The model under review builds one solid part; all positions refer to its coordinate system, in mm. A direction names the side the tool comes from. Round coordinates to 2 decimals unless told otherwise and drop trailing zeros. Write each loop counter-clockwise with the first axis right and the second up, starting at its lowest first coordinate (ties: lowest second). Pieces come first, ordered by that corner, then holes. Notation, with made-up numbers: (36, 83) -> (61, 83) arc R30 cw to (61, 121) -> close; hole circle Ø8 at (5.5, 86.5). An arc over 180 degrees is marked (long way). Return JSON: item names as keys, results as strings. Group by question number.
1. Take a section at A-A, the plane y = 15. Write out the cut boundary in (x, z).
2. For line 1 along X through (y, z) = (16.25, 0.5); line 2 along Z through (x, y) = (6.75, 18); line 3 along X through (y, z) = (8, -4.5), list the stretches that pass through material, from the lowest coordinate up. Write a range as from..to.
3. Take a section at B-B, the plane z = 0.25. Write out the cut boundary in (x, y), then the cut area to 3 significant figures.
4. Mouldability with a two-part tool opening along Y and no side actions: class faces 1 (the flat face through (2, 0, -1)), 2 (the flat face through (2, 20, -1)), 3 (the flat face through (6.252, 10, 2)) as pulls with the +Y half, pulls with the -Y half, needs draft (parallel to the pull), parting line crosses it, or undercut.
5. Clearance check with flat-ended pins moving along their axes: P1, Ø2, axis at y = 9, z = 3, coming from the -X side; P2, Ø2, axis at x = 8, y = 10.5, coming from the +Z side. State where each tip first meets the part, or that it passes through.
6. Take a section at C-C, the plane x = 9. Write out the cut boundary in (y, z), then the cut area to 3 significant figures.
7. Tool access review of faces 4 (the flat face through (8, 10, 0)), 5 (the flat face through (-1.748, 10, 2)), 6 (the flat face through (2, 10, -6.46)): name each direction out of +Z, -Z, +X, -X, +Y, -Y from which nothing blocks a thin tool from reaching the whole face with its end or side.
from build123d import *

# Parameters (mm, degrees)
BOSS_EXTRUDE1_DEPTH          = 40
SKETCH2_W                    = 3.5
SKETCH2_H                    = 40
BOSS_EXTRUDE2_DEPTH          = 5
SKETCH4_R                    = 2
CUT_EXTRUDE1_DEPTH           = 7
SKETCH5_R                    = 3.5
CUT_EXTRUDE2_DEPTH           = 3
CUT_EXTRUDE2_DRAFT           = -27
CUT_EXTRUDE2_PROFILE_2_DEPTH = 3
CUT_EXTRUDE2_PROFILE_2_DRAFT = -27
BOSS_EXTRUDE3_DEPTH          = 3
SKETCH9_W                    = 13
SKETCH9_H                    = 40
CUT_EXTRUDE4_DEPTH           = 4.702585656
SKETCH10_W                   = 15
SKETCH10_H                   = 40
BOSS_EXTRUDE4_DEPTH          = 2.5
SKETCH11_W                   = 1.5
SKETCH11_H                   = 2.202585656
BOSS_EXTRUDE7_DEPTH          = 40
BOSS_EXTRUDE8_DEPTH          = 0.625841469
SKETCH13_R                   = 2
CUT_EXTRUDE5_DEPTH           = 10
SKETCH14_W                   = 2.5
SKETCH14_H                   = 40
BOSS_EXTRUDE9_DEPTH          = 0.5
SKETCH15_W                   = 2.5
SKETCH15_H                   = 40
BOSS_EXTRUDE10_DEPTH         = 0.5
BOSS_EXTRUDE11_DEPTH         = 40
BOSS_EXTRUDE12_DEPTH         = 1.13137085
SKETCH18_R                   = 2
CUT_EXTRUDE6_DEPTH           = 10
SKETCH19_R                   = 3
CUT_EXTRUDE7_DEPTH           = 3
CUT_EXTRUDE7_DRAFT           = -19
CUT_EXTRUDE7_PROFILE_2_DEPTH = 3
CUT_EXTRUDE7_PROFILE_2_DRAFT = -19
SKETCH20_W                   = 5
SKETCH20_H                   = 40
BOSS_EXTRUDE13_DEPTH         = 0.5
SKETCH21_W                   = 5
SKETCH21_H                   = 40
BOSS_EXTRUDE14_DEPTH         = 0.5
SKETCH22_W                   = 7
SKETCH22_H                   = 6.5
SKETCH22_W_2                 = 7.5
CUT_EXTRUDE8_DEPTH           = 20
SKETCH23_R                   = 2
BOSS_EXTRUDE15_DEPTH         = 6.459797975
SKETCH24_R                   = 3
BOSS_EXTRUDE16_DEPTH         = 11.459797975
SKETCH25_W                   = 4
SKETCH25_H                   = 20
CUT_EXTRUDE9_DEPTH           = 20
SKETCH26_W                   = 8
SKETCH26_H                   = 20
CUT_EXTRUDE10_DEPTH          = 1


with BuildPart() as part:
    # Sketch1 → Boss-Extrude1 (new body)
    with BuildSketch(Plane(origin=(0, 0, 0), x_dir=(1, 0, 0), z_dir=(0, 1, 0))):
        Polygon((-4.247892457, 4.702585656), (8.752107543, 4.702585656), (8.752107543, 1.702585656), (7.049521887, 0), (-2.545306801, 0), (-4.247892457, 1.702585656), align=None)
    extrude(amount=BOSS_EXTRUDE1_DEPTH)

    # Sketch2 → Boss-Extrude2 (add)
    with BuildSketch(Plane.XY):
        with Locations((4.002107543, 20)):
            Rectangle(SKETCH2_W, SKETCH2_H)
        with Locations((0.502107543, 20)):
            Rectangle(SKETCH2_W, SKETCH2_H)
    extrude(amount=BOSS_EXTRUDE2_DEPTH)

    # Sketch4 → Cut-Extrude1 (cut)
    with BuildSketch(Plane.XY.offset(5)):
        with Locations((2.252107543, 30)):
            Circle(SKETCH4_R)
        with Locations((2.252107543, 10)):
            Circle(SKETCH4_R)
    extrude(amount=-CUT_EXTRUDE1_DEPTH, mode=Mode.SUBTRACT)


with BuildPart() as cut_extrude2_tool:
    # Sketch5 → Cut-Extrude2 (with draft: the straight prism first)
    with BuildSketch(Plane(origin=(0, 0, -4.702585656), x_dir=(-1, 0, 0), z_dir=(0, 0, -1))):
        with Locations((-2.252107543, 30)):
            Circle(SKETCH5_R)
    extrude(amount=-CUT_EXTRUDE2_DEPTH)
    # Cut-Extrude2: the draft: its side faces are tilted about the plane it starts from
    cut_extrude2_sides = [cut_extrude2_tool.faces().sort_by_distance(p)[0] for p in [
        (5.752107543, 30, -3.202585656),
    ]]
    draft(cut_extrude2_sides, Plane(origin=(0, 0, -4.702585656), x_dir=(-1, 0, 0), z_dir=(0, 0, -1)), CUT_EXTRUDE2_DRAFT)


with BuildPart() as part_1:
    add(part.part)

    # Cut-Extrude2: cut by cut_extrude2_tool
    add(cut_extrude2_tool.part, mode=Mode.SUBTRACT)


with BuildPart() as cut_extrude2_profile_2_tool:
    # Sketch5 → Cut-Extrude2 profile 2 (with draft: the straight prism first)
    with BuildSketch(Plane(origin=(0, 0, -4.702585656), x_dir=(-1, 0, 0), z_dir=(0, 0, -1))):
        with Locations((-2.252107543, 10)):
            Circle(SKETCH5_R)
    extrude(amount=-CUT_EXTRUDE2_PROFILE_2_DEPTH)
    # Cut-Extrude2 profile 2: the draft: its side faces are tilted about the plane it starts from
    cut_extrude2_profile_2_sides = [cut_extrude2_profile_2_tool.faces().sort_by_distance(p)[0] for p in [
        (5.752107543, 10, -3.202585656),
    ]]
    draft(cut_extrude2_profile_2_sides, Plane(origin=(0, 0, -4.702585656), x_dir=(-1, 0, 0), z_dir=(0, 0, -1)), CUT_EXTRUDE2_PROFILE_2_DRAFT)


with BuildPart() as part_2:
    add(part_1.part)

    # Cut-Extrude2 profile 2: cut by cut_extrude2_profile_2_tool
    add(cut_extrude2_profile_2_tool.part, mode=Mode.SUBTRACT)

    # Sketch7 → Boss-Extrude3 (add)
    with BuildSketch(Plane(origin=(0, 0, -4.702585656), x_dir=(-1, 0, 0), z_dir=(0, 0, -1))):
        Polygon((1.247892457, 46.5), (-5.752107543, 46.5), (-5.752107543, 40), (-4.252107543, 40), (-4.252107543, 45), (-0.252107543, 45), (-0.252107543, 43.275204256), (-0.252107543, 40), (1.247892457, 40), align=None)
        Polygon((-4.252107543, 0), (-5.752107543, 0), (-5.752107543, -6.5), (1.247892457, -6.5), (1.247892457, 0), (-0.252107543, 0), (-0.252107543, -5), (-4.252107543, -5), align=None)
    extrude(amount=-BOSS_EXTRUDE3_DEPTH)

    # Sketch9 → Cut-Extrude4 (cut)
    with BuildSketch(Plane(origin=(0, 0, -4.702585656), x_dir=(-1, 0, 0), z_dir=(0, 0, -1))):
        with Locations((-2.252107543, 20)):
            Rectangle(SKETCH9_W, SKETCH9_H)
    extrude(amount=-CUT_EXTRUDE4_DEPTH, mode=Mode.SUBTRACT)


with BuildPart() as cut_extrude4_piece_1:
    # of the separate pieces the step leaves, piece 1, a body of its own (cut_extrude4_pieces)
    add(part_2.part.solids().sort_by_distance((-1.247892457, 0, 0))[0])



with BuildPart() as cut_extrude4_piece_2:
    # of the separate pieces the step leaves, piece 2, a body of its own (cut_extrude4_pieces)
    add(part_2.part.solids().sort_by_distance((0.252107543, 40, -4.702585656))[0])


with BuildPart() as cut_extrude4_piece_3:
    # of the separate pieces the step leaves, piece 3, a body of its own (cut_extrude4_pieces)
    add(part_2.part.solids().sort_by_distance((-1.247892457, -6.5, -4.702585656))[0])


with BuildPart() as cut_extrude4_piece_1_1:
    add(cut_extrude4_piece_1.part)

    add(cut_extrude4_piece_2.part)  # Boss-Extrude4 merges Cut-Extrude4 piece 2

    add(cut_extrude4_piece_3.part)  # Boss-Extrude4 merges Cut-Extrude4 piece 3
    # Sketch10 → Boss-Extrude4 (add)
    with BuildSketch(Plane(origin=(0, 0, 0), x_dir=(-1, 0, 0), z_dir=(0, 0, -1))):
        with Locations((-2.252107543, 20)):
            Rectangle(SKETCH10_W, SKETCH10_H)
    extrude(amount=BOSS_EXTRUDE4_DEPTH)

    # Sketch11 → Boss-Extrude7 (add)
    with BuildSketch(Plane(origin=(0, 0, 0), x_dir=(1, 0, 0), z_dir=(0, 1, 0))):
        with Locations((5.002107543, 3.601292828)):
            Rectangle(SKETCH11_W, SKETCH11_H)
        Polygon((-2.419465332, 5.328427125), (-5.247892457, 2.5), (4.252107543, 2.5), (4.252107543, 4.702585656), (5.752107543, 4.702585656), (5.752107543, 2.5), (9.752107543, 2.5), (6.923680418, 5.328427125), align=None)
    extrude(amount=BOSS_EXTRUDE7_DEPTH)

    # Sketch12 → Boss-Extrude8 (add)
    with BuildSketch(Plane(origin=(0, 0, -4.702585656), x_dir=(-1, 0, 0), z_dir=(0, 0, -1))):
        Polygon((-5.752107543, 0), (-5.752107543, -6.5), (1.247892457, -6.5), (1.247892457, 0), (-0.252107543, 0), (-0.252107543, -5), (-4.252107543, -5), (-4.252107543, 0), align=None)
        Polygon((1.247892457, 46.5), (-5.752107543, 46.5), (-5.752107543, 40), (-4.252107543, 40), (-4.252107543, 45), (-0.252107543, 45), (-0.252107543, 40), (1.247892457, 40), align=None)
    extrude(amount=BOSS_EXTRUDE8_DEPTH)

    # Sketch13 → Cut-Extrude5 (cut)
    with BuildSketch(Plane.XY):
        with Locations((2.252107543, 30)):
            Circle(SKETCH13_R)
        with Locations((2.252107543, 10)):
            Circle(SKETCH13_R)
    extrude(amount=-CUT_EXTRUDE5_DEPTH, mode=Mode.SUBTRACT)

    # Sketch14 → Boss-Extrude9 (add)
    with BuildSketch(Plane(origin=(9.752107543, 0, 0), x_dir=(0, 0, -1), z_dir=(1, 0, 0))):
        with Locations((1.25, 20)):
            Rectangle(SKETCH14_W, SKETCH14_H)
    extrude(amount=BOSS_EXTRUDE9_DEPTH)

    # Sketch15 → Boss-Extrude10 (add)
    with BuildSketch(Plane.ZY.offset(5.247892457)):
        with Locations((-1.25, 20)):
            Rectangle(SKETCH15_W, SKETCH15_H)
    extrude(amount=BOSS_EXTRUDE10_DEPTH)

    # Sketch16 → Boss-Extrude11 (add)
    with BuildSketch(Plane.XZ):
        Polygon((-2.419465332, -5.328427125), (-5.247892457, -2.5), (-5.747892457, -2.5), (-5.747892457, -3.13137085), (-2.419465332, -6.459797975), (6.923680418, -6.459797975), (10.252107543, -3.13137085), (10.252107543, -2.5), (9.752107543, -2.5), (6.923680418, -5.328427125), (0.656985658, -5.328427125), align=None)
    extrude(amount=-BOSS_EXTRUDE11_DEPTH)

    # Sketch17 → Boss-Extrude12 (add)
    with BuildSketch(Plane(origin=(0, 0, -5.328427125), x_dir=(-1, 0, 0), z_dir=(0, 0, -1))):
        Polygon((-5.752107543, 0), (-5.752107543, -6.5), (1.247892457, -6.5), (1.247892457, 0), (0, 0), (0, -5), (-0.252107543, -5), (-4.252107543, -5), (-4.252107543, 0), align=None)
        Polygon((1.247892457, 46.5), (-5.752107543, 46.5), (-5.752107543, 40), (-4.252107543, 40), (-4.252107543, 44.953142187), (-0.252107543, 44.953142187), (-0.252107543, 40), (1.247892457, 40), align=None)
    extrude(amount=BOSS_EXTRUDE12_DEPTH)

    # Sketch18 → Cut-Extrude6 (cut)
    with BuildSketch(Plane.XY.offset(-5.328427125)):
        with Locations((2.252107543, 30)):
            Circle(SKETCH18_R)
        with Locations((2.252107543, 10)):
            Circle(SKETCH18_R)
    extrude(amount=-CUT_EXTRUDE6_DEPTH, mode=Mode.SUBTRACT)


with BuildPart() as cut_extrude7_tool:
    # Sketch19 → Cut-Extrude7 (with draft: the straight prism first)
    with BuildSketch(Plane(origin=(0, 0, -6.459797975), x_dir=(-1, 0, 0), z_dir=(0, 0, -1))):
        with Locations((-2.252107543, 30)):
            Circle(SKETCH19_R)
    extrude(amount=-CUT_EXTRUDE7_DEPTH)
    # Cut-Extrude7: the draft: its side faces are tilted about the plane it starts from
    cut_extrude7_sides = [cut_extrude7_tool.faces().sort_by_distance(p)[0] for p in [
        (5.252107543, 30, -4.959797975),
    ]]
    draft(cut_extrude7_sides, Plane(origin=(0, 0, -6.459797975), x_dir=(-1, 0, 0), z_dir=(0, 0, -1)), CUT_EXTRUDE7_DRAFT)


with BuildPart() as cut_extrude4_piece_1_2:
    add(cut_extrude4_piece_1_1.part)

    # Cut-Extrude7: cut by cut_extrude7_tool
    add(cut_extrude7_tool.part, mode=Mode.SUBTRACT)


with BuildPart() as cut_extrude7_profile_2_tool:
    # Sketch19 → Cut-Extrude7 profile 2 (with draft: the straight prism first)
    with BuildSketch(Plane(origin=(0, 0, -6.459797975), x_dir=(-1, 0, 0), z_dir=(0, 0, -1))):
        with Locations((-2.252107543, 10)):
            Circle(SKETCH19_R)
    extrude(amount=-CUT_EXTRUDE7_PROFILE_2_DEPTH)
    # Cut-Extrude7 profile 2: the draft: its side faces are tilted about the plane it starts from
    cut_extrude7_profile_2_sides = [cut_extrude7_profile_2_tool.faces().sort_by_distance(p)[0] for p in [
        (5.252107543, 10, -4.959797975),
    ]]
    draft(cut_extrude7_profile_2_sides, Plane(origin=(0, 0, -6.459797975), x_dir=(-1, 0, 0), z_dir=(0, 0, -1)), CUT_EXTRUDE7_PROFILE_2_DRAFT)


with BuildPart() as cut_extrude4_piece_1_3:
    add(cut_extrude4_piece_1_2.part)

    # Cut-Extrude7 profile 2: cut by cut_extrude7_profile_2_tool
    add(cut_extrude7_profile_2_tool.part, mode=Mode.SUBTRACT)

    # Sketch20 → Boss-Extrude13 (add)
    with BuildSketch(Plane.ZY.offset(1.247892457)):
        with Locations((2.5, 20)):
            Rectangle(SKETCH20_W, SKETCH20_H)
    extrude(amount=BOSS_EXTRUDE13_DEPTH)

    # Sketch21 → Boss-Extrude14 (add)
    with BuildSketch(Plane(origin=(5.752107543, 0, 0), x_dir=(0, 0, -1), z_dir=(1, 0, 0))):
        with Locations((-2.5, 20)):
            Rectangle(SKETCH21_W, SKETCH21_H)
    extrude(amount=BOSS_EXTRUDE14_DEPTH)

    # Sketch22 → Cut-Extrude8 (cut)
    with BuildSketch(Plane.XY.offset(5)):
        with Locations((2.252107543, 43.25)):
            Rectangle(SKETCH22_W, SKETCH22_H)
        with Locations((2.502107543, -3.25)):
            Rectangle(SKETCH22_W_2, SKETCH22_H)
    extrude(amount=-CUT_EXTRUDE8_DEPTH, mode=Mode.SUBTRACT)

    # Sketch23 → Boss-Extrude15 (add)
    with BuildSketch(Plane.XY):
        with Locations((2.252107543, 10)):
            Circle(SKETCH23_R)
        with Locations((2.252107543, 30)):
            Circle(SKETCH23_R)
    extrude(amount=-BOSS_EXTRUDE15_DEPTH)

    # Sketch24 → Boss-Extrude16 (add)
    with BuildSketch(Plane(origin=(0, 0, -6.459797975), x_dir=(-1, 0, 0), z_dir=(0, 0, -1))):
        with Locations((-2.252107543, 30)):
            Circle(SKETCH24_R)
        with Locations((-2.252107543, 10)):
            Circle(SKETCH24_R)
    extrude(amount=-BOSS_EXTRUDE16_DEPTH)

    # Sketch25 → Cut-Extrude9 (cut)
    with BuildSketch(Plane.XY.offset(5)):
        Polygon((6.252107543, 20.358230215), (6.252107543, 20), (10.252107543, 20), (10.252107543, 40), (6.252107543, 40), align=None)
        Polygon((-1.747892457, 20), (6.252107543, 20), (6.252107543, 20.358230215), (6.252107543, 40), (-1.747892457, 40), align=None)
        with Locations((-3.747892457, 30)):
            Rectangle(SKETCH25_W, SKETCH25_H)
    extrude(amount=-CUT_EXTRUDE9_DEPTH, mode=Mode.SUBTRACT)

    # Sketch26 → Cut-Extrude10 (cut)
    with BuildSketch(Plane.XY.offset(5)):
        with Locations((2.252107543, 10)):
            Rectangle(SKETCH26_W, SKETCH26_H)
    extrude(amount=-CUT_EXTRUDE10_DEPTH, mode=Mode.SUBTRACT)


solid = cut_extrude4_piece_1_3.part
Output:
{
 "1": {"outline": "(-5.75, -3.13) -> (-2.42, -6.46) -> (6.92, -6.46) -> (10.25, -3.13) -> (10.25, 0) -> (6.25, 0) -> (6.25, 4) -> (-1.75, 4) -> (-1.75, 0) -> (-5.75, 0) -> close"},
 "2": {"line 1": "x = -1.75..6.25", "line 2": "z = -6.46..0", "line 3": "x = -4.38..8.88"},
 "3": {"outline": "(-1.75, 0) -> (6.25, 0) -> (6.25, 20) -> (-1.75, 20) -> close", "area": "160 mm^2"},
 "4": {"face 1": "pulls with the -Y half", "face 2": "pulls with the +Y half", "face 3": "needs draft"},
 "5": {"P1": "stops at x = -1.75", "P2": "stops at z = 0"},
 "6": {"outline": "(0, -4.38) -> (20, -4.38) -> (20, 0) -> (0, 0) -> close", "area": "87.7 mm^2"},
 "7": {"face 4": "+Z, +X, +Y, -Y", "face 5": "+Z, -X, +Y, -Y", "face 6": "-Z, +X, -X, +Y, -Y"}
}
